```python
from build123d import *

# Parameters (mm, degrees)
SKETCH2_R           = 35
BOSS_EXTRUDE1_DEPTH = 25.4
CUT_EXTRUDE1_DEPTH  = 56.634162167
SKETCH5_R           = 2.1
CUT_EXTRUDE3_DEPTH  = 56.634162167


with BuildPart() as part:
    # Sketch2 → Boss-Extrude1 (new body)
    with BuildSketch(Plane(origin=(0, 0, 0), x_dir=(1, 0, 0), z_dir=(0, 1, 0))):
        with Locations(Location((0, 0, 0), (0, 0, 270))):
            Circle(SKETCH2_R)
    extrude(amount=BOSS_EXTRUDE1_DEPTH)

    # Sketch3 → Cut-Extrude1 (cut, through all)
    with BuildSketch(Plane(origin=(0, 25.4, 0), x_dir=(1, 0, 0), z_dir=(0, 1, 0))):
        with BuildLine():
            ThreePointArc((-1.658312395, 2.5), (0, -3), (1.658312395, 2.5))
            ThreePointArc((1.658312395, 2.5), (0, 3), (-1.658312395, 2.5))
        make_face()
    extrude(amount=-CUT_EXTRUDE1_DEPTH, mode=Mode.SUBTRACT)

    # Sketch5 → Cut-Extrude3 (cut, through all)
    with BuildSketch(Plane(origin=(0, 25.4, 0), x_dir=(1, 0, 0), z_dir=(0, 1, 0))):
        with Locations(Location((0, 25, 0), (0, 0, 270))):
            Circle(SKETCH5_R)
        with Locations(Location((21.650635095, 12.5, 0), (0, 0, 270))):
            Circle(SKETCH5_R)
        with Locations(Location((21.650635095, -12.5, 0), (0, 0, 270))):
            Circle(SKETCH5_R)
        with Locations(Location((0, -25, 0), (0, 0, 270))):
            Circle(SKETCH5_R)
        with Locations(Location((-21.650635095, -12.5, 0), (0, 0, 270))):
            Circle(SKETCH5_R)
        with Locations(Location((-21.650635095, 12.5, 0), (0, 0, 270))):
            Circle(SKETCH5_R)
    extrude(amount=-CUT_EXTRUDE3_DEPTH, mode=Mode.SUBTRACT)


solid = part.part
```
Design review of the part built by this model. Coordinates are the model's own, in mm. Round coordinates to 2 decimals unless told otherwise and drop trailing zeros. Write each loop counter-clockwise with the first axis right and the second up, starting at its lowest first coordinate (ties: lowest second). Pieces come first, ordered by that corner, then holes. Notation, with made-up numbers: (5.25, 17) -> (52.25, 17) arc R12 cw to (52.25, 30) -> close; hole circle Ø5 at (47.5, 60.25). An arc over 180 degrees is marked (long way). Answer in a Markdown table with one row per item.
Q1. Take a section at B-B, the plane z = 0. State the section outline as (x, y) points.
The answers:
| item | result |
|---|---|
| outline | (-35, 0) -> (-3, 0) -> (-3, 25.4) -> (-35, 25.4) -> close; (3, 0) -> (35, 0) -> (35, 25.4) -> (3, 25.4) -> close |
Q2. Take a section at C-C, the plane y = 23.25. State the section outline as (x, z) points, then the cut area to 3 significant figures.
The answers:
| item | result |
|---|---|
| outline | circle Ø70 at (0, 0); hole circle Ø4.2 at (-21.65, -12.5); hole circle Ø4.2 at (-21.65, 12.5); hole circle Ø6 at (0, 0); hole circle Ø4.2 at (0, -25); hole circle Ø4.2 at (0, 25); hole circle Ø4.2 at (21.65, -12.5); hole circle Ø4.2 at (21.65, 12.5) |
| area | 3,740 mm² |
Q3. Take a section at D-D, the plane z = 12.5. State the section outline as (x, y) points, then the cut area to 3 significant figures.
The answers:
| item | result |
|---|---|
| outline | (-32.69, 0) -> (-23.75, 0) -> (-23.75, 25.4) -> (-32.69, 25.4) -> close; (-19.55, 0) -> (19.55, 0) -> (19.55, 25.4) -> (-19.55, 25.4) -> close; (23.75, 0) -> (32.69, 0) -> (32.69, 25.4) -> (23.75, 25.4) -> close |
| area | 1,450 mm² |
Q4. Draft analysis for pull direction Z (two halves, no side actions). For faces 1 (the face through (-21, 13, -28)), 2 (the face through (0, 0, 7)), 3 (the face through (-0.8, 12.88, 26.94)), state which applies: +Z half, -Z half, draft (parallel to the pull), parting line (faces both ways), or undercut.
The answers:
| item | result |
|---|---|
| face 1 | parting line |
| face 2 | draft |
| face 3 | undercut |
Q5. Clearance check with flat-ended pins moving along their axes: pin 1 Ø5 at (y, z) = (19, 19) entering from -X; pin 2 Ø4 at (x, y) = (25.5, 9.5) entering from -Z; pin 3 Ø4 at (y, z) = (13.5, -8.5) entering from -X. State where each tip first meets the part, or that it passes through.
The answers:
| item | result |
|---|---|
| pin 1 | x = -30.87 |
| pin 2 | z = -25.94 |
| pin 3 | x = -34.39 |
Q6. Take a section at A-A, the plane x = 0. State the section outline as (y, z) points, then the cut area to 3 significant figures.
The answers:
| item | result |
|---|---|
| outline | (0, -35) -> (25.4, -35) -> (25.4, -27.1) -> (0, -27.1) -> close; (0, -22.9) -> (25.4, -22.9) -> (25.4, -3) -> (0, -3) -> close; (0, 3) -> (25.4, 3) -> (25.4, 22.9) -> (0, 22.9) -> close; (0, 27.1) -> (25.4, 27.1) -> (25.4, 35) -> (0, 35) -> close |
| area | 1,410 mm² |
Q7. To check wall thickness, follow L1, parallel to Z at x = -0.5, y = 14.25; L2, parallel to X at y = 12.25, z = 13.5; L3, parallel to Z at x = 20, y = 7.5. State the ranges of each line that lie inside material, in increasing order. Write a range as [from, to].
The answers:
| item | result |
|---|---|
| L1 | [-35, -27.04], [-22.96, -2.96], [2.96, 22.96], [27.04, 35] |
| L2 | [-32.29, -23.5], [-19.8, 19.8], [23.5, 32.29] |
| L3 | [-28.72, -13.8], [-11.2, 11.2], [13.8, 28.72] |
